from build123d import *

# Parameters (mm, degrees)
SKETCH2_R               = 50.8
SKETCH2_R_2             = 41.275
BASE_CYLINDER_DEPTH     = 292.1
SKETCH3_R               = 69.85
SKETCH3_R_2             = 41.275
AFT_FLANGE_DEPTH        = 12.7
SKETCH4_R               = 69.85
SKETCH4_R_2             = 41.275
FORWARD_FLANGE_DEPTH    = 12.7
SKETCH6_R               = 49.53
SKETCH6_R_2             = 47.625
O_RING_SLOT_1_DEPTH     = 1.1176
SKETCH7_R               = 49.53
SKETCH7_R_2             = 47.625
O_RING_SLOT_2_DEPTH     = 1.1176
SKETCH8_R               = 3.175
CUT_EXTRUDE4_DEPTH      = 1
CUT_EXTRUDE4_DEPTH_BACK = 293.1


with BuildPart() as part:
    # Sketch2 → Base Cylinder (new body)
    with BuildSketch(Plane(origin=(0, 0, 0), x_dir=(1, 0, 0), z_dir=(0, 1, 0))):
        Circle(SKETCH2_R)
        Circle(SKETCH2_R_2, mode=Mode.SUBTRACT)
    extrude(amount=BASE_CYLINDER_DEPTH)

    # Sketch3 → Aft Flange (add)
    with BuildSketch(Plane.XZ):
        Circle(SKETCH3_R)
        Circle(SKETCH3_R_2, mode=Mode.SUBTRACT)
    extrude(amount=-AFT_FLANGE_DEPTH)

    # Sketch4 → Forward Flange (add)
    with BuildSketch(Plane(origin=(0, 292.1, 0), x_dir=(1, 0, 0), z_dir=(0, 1, 0))):
        Circle(SKETCH4_R)
        Circle(SKETCH4_R_2, mode=Mode.SUBTRACT)
    extrude(amount=-FORWARD_FLANGE_DEPTH)

    # Sketch6 → O-Ring Slot 1 (cut)
    with BuildSketch(Plane.XZ):
        Circle(SKETCH6_R)
        Circle(SKETCH6_R_2, mode=Mode.SUBTRACT)
    extrude(amount=-O_RING_SLOT_1_DEPTH, mode=Mode.SUBTRACT)

    # Sketch7 → O-Ring Slot 2 (cut)
    with BuildSketch(Plane(origin=(0, 292.1, 0), x_dir=(1, 0, 0), z_dir=(0, 1, 0))):
        Circle(SKETCH7_R)
        Circle(SKETCH7_R_2, mode=Mode.SUBTRACT)
    extrude(amount=-O_RING_SLOT_2_DEPTH, mode=Mode.SUBTRACT)

    # Sketch8 → Cut-Extrude4 (cut, two sides)
    with BuildSketch(Plane.XZ) as cut_extrude4_sk:
        with Locations((-59.9186, 0)):
            Circle(SKETCH8_R)
        with Locations((-42.368848379, 42.368848379)):
            Circle(SKETCH8_R)
        with Locations((0, 59.9186)):
            Circle(SKETCH8_R)
        with Locations((42.368848379, 42.368848379)):
            Circle(SKETCH8_R)
        with Locations((59.9186, 0)):
            Circle(SKETCH8_R)
        with Locations((42.368848379, -42.368848379)):
            Circle(SKETCH8_R)
        with Locations((0, -59.9186)):
            Circle(SKETCH8_R)
        with Locations((-42.368848379, -42.368848379)):
            Circle(SKETCH8_R)
    extrude(amount=CUT_EXTRUDE4_DEPTH, mode=Mode.SUBTRACT)
    extrude(cut_extrude4_sk.sketch, amount=-CUT_EXTRUDE4_DEPTH_BACK, mode=Mode.SUBTRACT)


solid = part.part
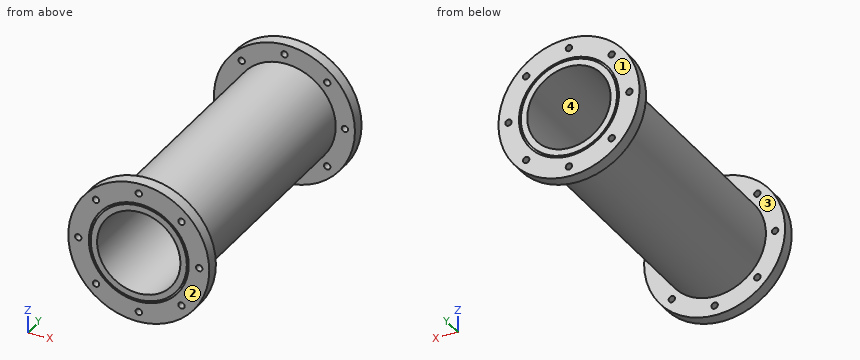
Source: CAD feature listing. Evaluate the final solid. Frame: model axes, mm. Face numbers are marked on the shaded views. Give positions to 0.01 mm unless a question says otherwise; leave off trailing zeros. Write each loop counter-clockwise with the first axis right and the second up, starting at its lowest first coordinate (ties: lowest second). Pieces come first, ordered by that corner, then holes. Notation, with made-up numbers: M 75,-19 L 79,-19 A21 ccw 79,11 Z; hole C 2,-5 d6. An arc over 180 degrees is marked long. Answer as a JSON object with one key per item and string values.
Q1. Cut plane D-D, the plane x = 0. Count the separate pieces of the cut face and the enclosed holes in it, then the cut area to 3 significant figures.
Geometry check:
{"separate pieces": "6", "enclosed holes": "0", "area": "6,200 mm^2"}
Q2. Contact query for flat-ended pins moving along their axis: P1, Ø12, axis at x = 42.5, y = 49.5, coming from the +Z side; P2, Ø6, axis at x = -39, y = 249.5, coming from the +Z side; P3, Ø5, axis at x = 0, z = -59.92, coming from the +Y side; P4, Ø6, axis at x = -38, y = 133.5, coming from the -Z side. Output: stop coordinate, or through.
Geometry check:
{"P1": "stops at z = 35.33", "P2": "stops at z = 35.84", "P3": "passes through", "P4": "stops at z = -36.82"}
Q3. Mould query, pull axis Y, two halves, no side actions, for the marked faces 1, 2, 3 and 4. Classes: +Y half, -Y half, draft (parallel to the pull), parting line (faces both ways), or undercut.
Geometry check:
{"face 1": "+Y half", "face 2": "-Y half", "face 3": "undercut", "face 4": "draft"}
Q4. Cut plane C-C, the plane y = 153. Return the cut outline in (x, z) (3 decimals), then the cut area to 3 significant figures.
Geometry check:
{"outline": "C 0,0 d101.6; hole C 0,0 d82.55", "area": "2,760 mm^2"}
Q5. Ray query, line 1 along Y through (x, z) = (48, 40); line 2 along X through (y, z) = (235.5, 3.5); line 3 along X through (y, z) = (141.5, 36.5). Return the intervals inside material, ascending.
Geometry check:
{"line 1": "y = 0 to 12.7, 279.4 to 292.1", "line 2": "x = -50.68 to -41.13, 41.13 to 50.68", "line 3": "x = -35.33 to -19.27, 19.27 to 35.33"}
